Verification items for the finished model (mm, model axes). A direction names the side the tool comes from. Round coordinates to 2 decimals unless told otherwise and drop trailing zeros. Write each loop counter-clockwise with the first axis right and the second up, starting at its lowest first coordinate (ties: lowest second). Pieces come first, ordered by that corner, then holes. Notation, with made-up numbers: M 33,-15 L 68,-15 A20 cw 68,-3 Z; hole C 89.25,73.25 d10. An arc over 180 degrees is marked long. One line per question, with ' | ' between items.
from build123d import *

# Parameters (mm, degrees)
BOSS_EXTRUDE1_DEPTH   = 36.425
CUT_EXTRUDE1_DEPTH    = 110.090212662
CUT_EXTRUDE2_DEPTH    = 109.098783751
FILLET1_R             = 4
BOSS_EXTRUDE14_START  = 25.3
BOSS_EXTRUDE14_DEPTH  = 2
CUT_EXTRUDE10_DEPTH   = 5
FILLET13_R            = 4
FILLET14_R            = 2
FILLET13_OF_MIRROR1_R = 4
FILLET14_OF_MIRROR1_R = 2


with BuildPart() as part:
    # Sketch1 → Boss-Extrude1 (new, symmetric)
    with BuildSketch(Plane.XY):
        with BuildLine():
            Line((0, 0), (-17.110884891, -59.672747116))
            ThreePointArc((-17.110884891, -59.672747116), (-22.347799076, -68.454296451), (-31.240591359, -73.5))
            Line((-31.240591359, -73.5), (-30.858426801, -74.9505))
            ThreePointArc((-30.858426801, -74.9505), (-21.298675096, -69.526368685), (-15.668992347, -60.08620315))
            Line((-15.668992347, -60.08620315), (1.441892544, -0.413456034))
            Line((1.441892544, -0.413456034), (1.560449154, 0))
            Line((1.560449154, 0), (0, 0))
        make_face()
    extrude(amount=BOSS_EXTRUDE1_DEPTH, both=True)

    # Sketch2 → Cut-Extrude1 (cut, through all)
    with BuildSketch(Plane.XY.offset(36.425)):
        with BuildLine():
            Line((-31.240591359, -73.5), (-26.943866684, -73.5))
            ThreePointArc((-26.943866684, -73.5), (-28.865857957, -74.320486174), (-30.858426801, -74.9505))
            Line((-30.858426801, -74.9505), (-31.240591359, -73.5))
        make_face()
    extrude(amount=-CUT_EXTRUDE1_DEPTH, mode=Mode.SUBTRACT)

    # Sketch3 → Cut-Extrude2 (cut, through all)
    with BuildSketch(Plane.XY.offset(36.425)):
        with BuildLine():
            Line((-26.943866684, -73.5), (-31.240591359, -73.5))
            ThreePointArc((-31.240591359, -73.5), (-29.043541661, -72.783058785), (-26.943866684, -71.817451685))
            Line((-26.943866684, -71.817451685), (-26.943866684, -73.5))
        make_face()
    extrude(amount=-CUT_EXTRUDE2_DEPTH, mode=Mode.SUBTRACT)

    # Fillet1
    fillet1_edges = [part.edges().sort_by_distance(p)[0] for p in [
        (0.780224577, 0, 36.425),
        (0.780224577, 0, -36.425),
    ]]
    fillet(fillet1_edges, radius=FILLET1_R)

    # Sketch33 → Boss-Extrude14 (add)
    with BuildSketch(Plane.XY.offset(BOSS_EXTRUDE14_START)):
        Polygon((-0.573490772, -2), (-9.867453858, -2), (-9.867453858, -10), (-2.867453858, -10), align=None)
    boss_extrude14 = extrude(amount=-BOSS_EXTRUDE14_DEPTH)

    # Sketch34 → Cut-Extrude10 (cut)
    with BuildSketch(Plane.XY.offset(25.3)):
        with BuildLine():
            ThreePointArc((-2.090857418, -3.811861892), (-3.261138108, -3.017857418), (-4.055142582, -4.188138108))
            ThreePointArc((-4.055142582, -4.188138108), (-4.865186914, -6.338616825), (-7.148892582, -6.594388108))
            ThreePointArc((-7.148892582, -6.594388108), (-8.478611892, -7.075892582), (-7.997107418, -8.405611892))
            ThreePointArc((-7.997107418, -8.405611892), (-3.637305687, -7.91732126), (-2.090857418, -3.811861892))
        make_face()
    cut_extrude10 = extrude(amount=-CUT_EXTRUDE10_DEPTH, mode=Mode.SUBTRACT)

    # Fillet13
    fillet13_edges = [part.edges().sort_by_distance(p)[0] for p in [
        (-9.867453858, -2, 24.3),
    ]]
    fillet(fillet13_edges, radius=FILLET13_R)

    # Fillet14
    fillet14_edges = [part.edges().sort_by_distance(p)[0] for p in [
        (-9.867453858, -10, 24.3),
    ]]
    fillet(fillet14_edges, radius=FILLET14_R)

    # Mirror1: Boss-Extrude14, Cut-Extrude10 across plane
    add(boss_extrude14.mirror(Plane.XY))
    add(cut_extrude10.mirror(Plane.XY), mode=Mode.SUBTRACT)

    # Fillet13 of Mirror1
    fillet13_of_mirror1_edges = [part.edges().sort_by_distance(p)[0] for p in [
        (-9.867453858, -2, -24.3),
    ]]
    fillet(fillet13_of_mirror1_edges, radius=FILLET13_OF_MIRROR1_R)

    # Fillet14 of Mirror1
    fillet14_of_mirror1_edges = [part.edges().sort_by_distance(p)[0] for p in [
        (-9.867453858, -10, -24.3),
    ]]
    fillet(fillet14_of_mirror1_edges, radius=FILLET14_OF_MIRROR1_R)


solid = part.part
1. Section check B-B, the plane x = -22.75. Record the cut outline in (y, z) (3 decimals).
Results:
outline: M -70.823,-36.425 L -68.837,-36.425 L -68.837,36.425 L -70.823,36.425 Z
2. Thickness scan on line 1 (Y direction, x = -18, z = 19); line 2 (X direction, y = -19.5, z = -18.5); line 3 (Y direction, x = -20.75, z = 21). Record the ranges inside material, lowest first.
Results:
line 1: y = -65.39 to -62.15 | line 2: x = -5.59 to -4.03 | line 3: y = -68.97 to -66.69
3. Section check A-A, the plane z = 3. Record the cut outline in (x, y), then the cut area to 3 significant figures.
Results:
outline: M -26.94,-73.5 A21.5 ccw -15.67,-60.09 L 1.56,0 L 0,0 L -17.11,-59.67 A20 cw -26.94,-71.82 Z | area: 119 mm2
4. Section check C-C, the plane y = -54. Record the cut outline in (x, z) (3 decimals).
Results:
outline: M -15.484,-36.425 L -13.924,-36.425 L -13.924,36.425 L -15.484,36.425 Z
5. Go/stop test with flat-tipped pins: P1, Ø1, axis at x = -4.5, z = 24, coming from the +Y side; P2, Ø2.5, axis at x = -3.5, y = -6, coming from the +Z side; P3, Ø1, axis at x = -21.5, z = -5, coming from the -Y side. Record where each tip stops, or that it passes through.
Results:
P1: stops at y = -2 | P2: stops at z = 25.3 | P3: stops at y = -70.18
6. Mould release check, pull along Y, two halves, no side actions. Record for faces 1 (the face through (-3, -2, 24)), 2 (the face through (-5, -10, 24)), 3 (the face through (-6, -5, -25.3)): pulls with the +Y half, pulls with the -Y half, needs draft (parallel to the pull), parting line crosses it, or undercut.
Results:
face 1: pulls with the +Y half | face 2: undercut | face 3: needs draft
7. Tool access check on faces 4 (the face through (-6, -5, 25.3)), 5 (the face through (-5, -10, -24)), 6 (the face through (-3, -2, -24)). Record the directions out of +Z, -Z, +X, -X, +Y, -Y that give a thin tool (end or side, any length) a straight path to the whole face; none if there is none.
Results:
face 4: +Z, -X, +Y | face 5: +Z, -Z, -X | face 6: +Z, -Z, -X, +Y
